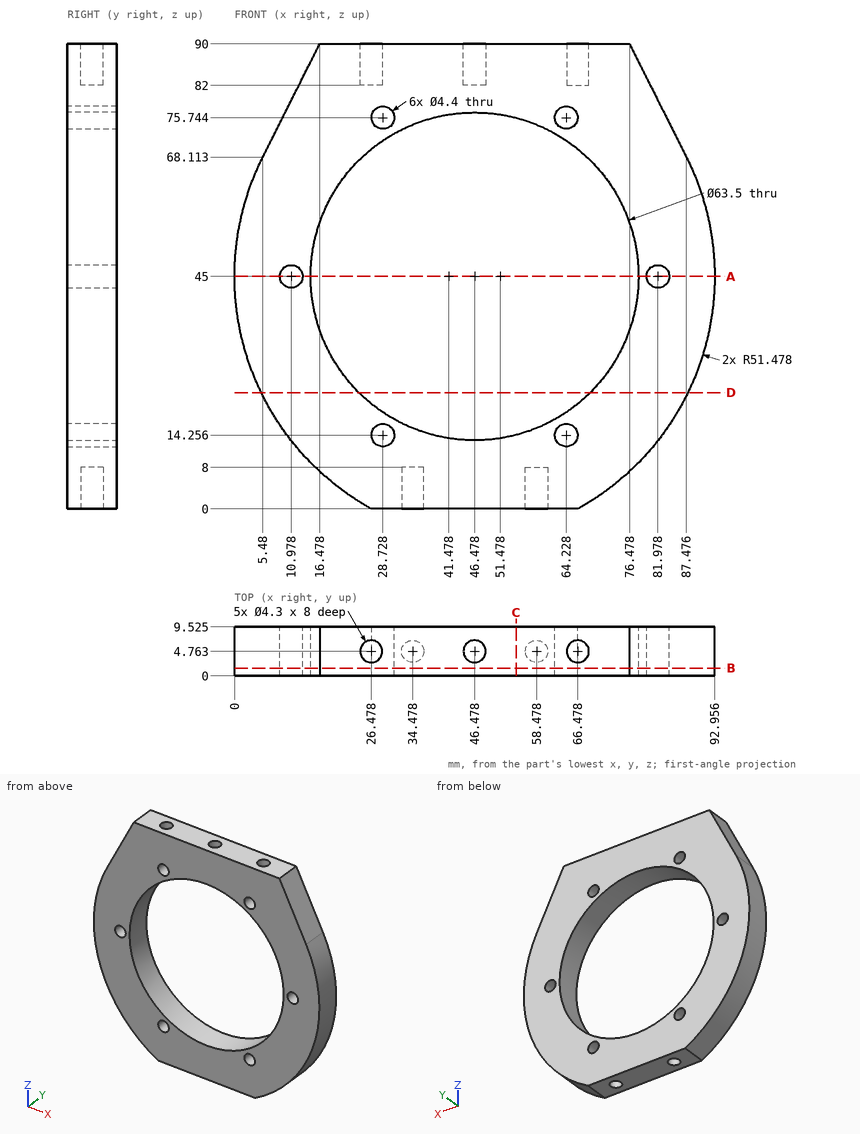
Answer from the drawing. Dimensions are ordinates in mm from the lowest x, y and z of the part. Coordinates: 2 decimals unless noted, no trailing zeros. Write each loop counter-clockwise with the first axis right and the second up, starting at its lowest first coordinate (ties: lowest second). Pieces come first, ordered by that corner, then holes. Notation, with made-up numbers: M -21,68 L 22,68 A26 ccw 22,100 Z; hole C 24.25,41 d5. An arc over 180 degrees is marked long. Use a Markdown table: item, result.
Q1. The part is cut by section D-D, the plane z = 22.5. Write down the section's boundary in (x, y) (1 decimal), then the cut area to 3 significant figures.
Answer block:
| item | result |
|---|---|
| outline | M 5.2,0 L 24.1,0 L 24.1,9.5 L 5.2,9.5 Z; M 68.9,0 L 87.8,0 L 87.8,9.5 L 68.9,9.5 Z |
| area | 360 mm2 |
Q2. The part is cut by section C-C, the plane x = 54.5. Write down the section's boundary in (y, z) (1 decimal).
Answer block:
| item | result |
|---|---|
| outline | M 0,0 L 9.5,0 L 9.5,14.3 L 0,14.3 Z; M 0,75.7 L 9.5,75.7 L 9.5,90 L 0,90 Z |
Q3. The part is cut by section A-A, the plane z = 45. Write down the section's boundary in (x, y) (1 decimal), then the cut area to 3 significant figures.
Answer block:
| item | result |
|---|---|
| outline | M 0,0 L 8.8,0 L 8.8,9.5 L 0,9.5 Z; M 13.2,0 L 14.7,0 L 14.7,9.5 L 13.2,9.5 Z; M 78.2,0 L 79.8,0 L 79.8,9.5 L 78.2,9.5 Z; M 84.2,0 L 93,0 L 93,9.5 L 84.2,9.5 Z |
| area | 197 mm2 |
Q4. Each of these flat-tipped pins is pushed along its axis until it touches: pin 1 Ø2 at (x, y) = (46.5, 5) entering from +Z; pin 2 Ø2.5 at (x, y) = (58.48, 4.76) entering from -Z; pin 3 Ø4 at (x, y) = (80.5, 8.5) entering from +Z (1 decimal). Where does it stop, or does it pass through?
Answer block:
| item | result |
|---|---|
| pin 1 | stops at z = 82 |
| pin 2 | stops at z = 8 |
| pin 3 | stops at z = 86 |
Q5. Straight lines are drawn through the part: L1, parallel to X at y = 4, z = 45; L2, parallel to Z at x = 9.5, y = 1 (1 decimal); L3, parallel to Z at x = 69, y = 8.25 (1 decimal). For each, find the intervals that lie inside material, in ascending order. Write a range as [from, to].
Answer block:
| item | result |
|---|---|
| L1 | x = [0, 8.78], [13.18, 14.73], [78.23, 79.78], [84.18, 92.96] |
| L2 | z = [15.2, 43.4], [46.6, 76.1] |
| L3 | z = [1.5, 22.6], [67.4, 90] |
Q6. The part is cut by section B-B, the plane y = 1.5. Give the number of separate pieces and of enclosed holes in the cut face.
Answer block:
| item | result |
|---|---|
| separate pieces | 1 |
| enclosed holes | 7 |
